```python
from build123d import *

# Parameters (mm, degrees)
SKETCH1_W           = 177.8
SKETCH1_H           = 88.9
BOSS_EXTRUDE1_DEPTH = 69.85
SHELL1_T            = -4.7625
SKETCH3_R           = 36
CUT_EXTRUDE1_DEPTH  = 57.912
SKETCH4_R           = 2.7
CUT_EXTRUDE4_DEPTH  = 3
SKETCH5_W           = 3.175
SKETCH5_H           = 58.95074776
BOSS_EXTRUDE4_DEPTH = 13.208
SKETCH8_W           = 1.447073232
SKETCH8_H           = 1.651
CUT_EXTRUDE8_DEPTH  = 56.134


with BuildPart() as part:
    # Sketch1 → Boss-Extrude1 (new body)
    with BuildSketch(Plane(origin=(0, 0, 0), x_dir=(1, 0, 0), z_dir=(0, 1, 0))):
        Rectangle(SKETCH1_W, SKETCH1_H)
    extrude(amount=BOSS_EXTRUDE1_DEPTH)

    # Shell1
    shell1_openings = [part.faces().sort_by_distance(p)[0] for p in [
        (0, 34.925, 44.45),
    ]]
    offset(amount=SHELL1_T, openings=shell1_openings, kind=Kind.INTERSECTION)

    # Sketch3 → Cut-Extrude1 (cut)
    with BuildSketch(Plane(origin=(0, 69.85, 0), x_dir=(1, 0, 0), z_dir=(0, 1, 0))):
        with Locations(Location((0, 0, 0), (0, 0, 270))):
            Circle(SKETCH3_R)
    extrude(amount=-CUT_EXTRUDE1_DEPTH, mode=Mode.SUBTRACT)

    # Sketch4 → Cut-Extrude4 (cut)
    with BuildSketch(Plane(origin=(0, 69.85, 0), x_dir=(1, 0, 0), z_dir=(0, 1, 0))):
        with Locations(Location((-31.373598792, 31.373598792, 0), (0, 0, 270))):
            Circle(SKETCH4_R)
        with Locations(Location((31.373598792, 31.373598792, 0), (0, 0, 90))):
            Circle(SKETCH4_R)
        with Locations(Location((31.373598792, -31.373598792, 0), (0, 0, 270))):
            Circle(SKETCH4_R)
        with Locations(Location((-31.373598792, -31.373598792, 0), (0, 0, 90))):
            Circle(SKETCH4_R)
    extrude(amount=-CUT_EXTRUDE4_DEPTH, mode=Mode.SUBTRACT)

    # Sketch5 → Boss-Extrude4 (add)
    with BuildSketch(Plane(origin=(0, 4.7625, 0), x_dir=(1, 0, 0), z_dir=(0, 1, 0))):
        with Locations((-2.654293776, -11.925687975)):
            Rectangle(SKETCH5_W, SKETCH5_H)
        Polygon((-69.646793776, -41.401061855), (-69.646793776, 17.549685905), (-72.821793776, 17.549685905), (-72.821793776, 0), (-72.821793776, -41.401061855), align=None)
    extrude(amount=BOSS_EXTRUDE4_DEPTH)

    # Sketch8 → Cut-Extrude8 (cut)
    with BuildSketch(Plane.XY.offset(41.401061855)):
        with Locations((-70.370330392, 10.16)):
            Rectangle(SKETCH8_W, SKETCH8_H)
        with Locations((-3.51825716, 10.16)):
            Rectangle(SKETCH8_W, SKETCH8_H)
    extrude(amount=-CUT_EXTRUDE8_DEPTH, mode=Mode.SUBTRACT)


solid = part.part
```
Geometry: final body of the model. Coordinates: model frame, mm. A direction names the side the tool comes from. Round coordinates to 2 decimals unless told otherwise and drop trailing zeros. Write each loop counter-clockwise with the first axis right and the second up, starting at its lowest first coordinate (ties: lowest second). Pieces come first, ordered by that corner, then holes. Notation, with made-up numbers: M 51,-2 L 107,-2 A11 cw 107,2 Z; hole C 53.25,-40 d3. An arc over 180 degrees is marked long. Answer in a Markdown table with one row per item. Add a question column.
(1) Draft query along Y for faces 4 (the face through (-21, 69.85, -30)), 5 (the face through (-72.822, 11, 12)), 6 (the face through (32, 68, -34)). Return one class per face: pulls with the +Y half, pulls with the -Y half, needs draft (parallel to the pull), parting line crosses it, or undercut.
(2) Ray query, L1, parallel to X at y = 10, z = 34.5; L2, parallel to X at y = 13, z = 24; L3, parallel to X at y = 67.55, z = 0. Return the intervals inside material, ascending.
(3) Reachability of faces 1 (the face through (30.34, 68.37, 33.87)), 2 (the face through (-71, 11, -17.55)), 3 (the face through (-1, 65.087, 39)) from +Z, -Z, +X, -X, +Y, -Y: full face, straight path, thin tool, end or side. Return the list, or none.
(4) Cut plane B-B, the plane y = 38. Return the cut outline in (x, z), then the cut area to 3 significant figures.
(5) Cut plane C-C, the plane z = 0. Return the cut outline in (x, y), then the cut area to 3 significant figures.
(6) Cut plane D-D, the plane z = 21.5. Return the cut outline in (x, y), then the cut area to 3 significant figures.
(7) Cut plane A-A, the plane x = -57.5. Return the cut outline in (y, z), then the cut area to 3 significant figures.
(8) Contact query for flat-ended pins moving along their axis: pin 1 (0.7 mm diameter, centred on x = -70.5, y = 10, fed in from +Z); pin 2 (5 mm diameter, centred on x = 31.37, z = -31.37, fed in from +Y); pin 3 (2.5 mm diameter, centred on x = -3, z = 5, fed in from +Y); pin 4 (6 mm diameter, centred on x = -31.37, z = -31.37, fed in from -Y). Output: stop coordinate, or through.
Established:
| question | item | result |
|---|---|---|
| 1 | face 4 | pulls with the +Y half |
| 1 | face 5 | undercut |
| 1 | face 6 | needs draft |
| 2 | L1 | -88.9 to -84.14, -72.82 to -71.09, -2.79 to -1.07, 84.14 to 88.9 |
| 2 | L2 | -88.9 to -84.14, -72.82 to -69.65, -4.24 to -1.07, 84.14 to 88.9 |
| 2 | L3 | -88.9 to -36, 36 to 88.9 |
| 3 | face 1 | +Y |
| 3 | face 2 | none |
| 3 | face 3 | +Z |
| 4 | outline | M -88.9,-44.45 L 88.9,-44.45 L 88.9,44.45 L 84.14,44.45 L 84.14,-39.69 L -84.14,-39.69 L -84.14,44.45 L -88.9,44.45 Z |
| 4 | area | 1,650 mm² |
| 5 | outline | M -88.9,0 L 88.9,0 L 88.9,69.85 L 36,69.85 L 36,65.09 L 84.14,65.09 L 84.14,4.76 L -1.07,4.76 L -1.07,17.97 L -4.24,17.97 L -4.24,10.99 L -2.79,10.99 L -2.79,9.33 L -4.24,9.33 L -4.24,4.76 L -69.65,4.76 L -69.65,9.33 L -71.09,9.33 L -71.09,10.99 L -69.65,10.99 L -69.65,17.97 L -72.82,17.97 L -72.82,4.76 L -84.14,4.76 L -84.14,65.09 L -36,65.09 L -36,69.85 L -88.9,69.85 Z |
| 5 | area | 2,000 mm² |
| 6 | outline | M -88.9,0 L 88.9,0 L 88.9,69.85 L 28.87,69.85 L 28.87,65.09 L 84.14,65.09 L 84.14,4.76 L -1.07,4.76 L -1.07,17.97 L -4.24,17.97 L -4.24,10.99 L -2.79,10.99 L -2.79,9.33 L -4.24,9.33 L -4.24,4.76 L -69.65,4.76 L -69.65,9.33 L -71.09,9.33 L -71.09,10.99 L -69.65,10.99 L -69.65,17.97 L -72.82,17.97 L -72.82,4.76 L -84.14,4.76 L -84.14,65.09 L -28.87,65.09 L -28.87,69.85 L -88.9,69.85 Z |
| 6 | area | 2,070 mm² |
| 7 | outline | M 0,-44.45 L 69.85,-44.45 L 69.85,44.45 L 65.09,44.45 L 65.09,-39.69 L 4.76,-39.69 L 4.76,44.45 L 0,44.45 Z |
| 7 | area | 1,130 mm² |
| 8 | pin 1 | z = -14.73 |
| 8 | pin 2 | y = 66.85 |
| 8 | pin 3 | y = 17.97 |
| 8 | pin 4 | y = 0 |
